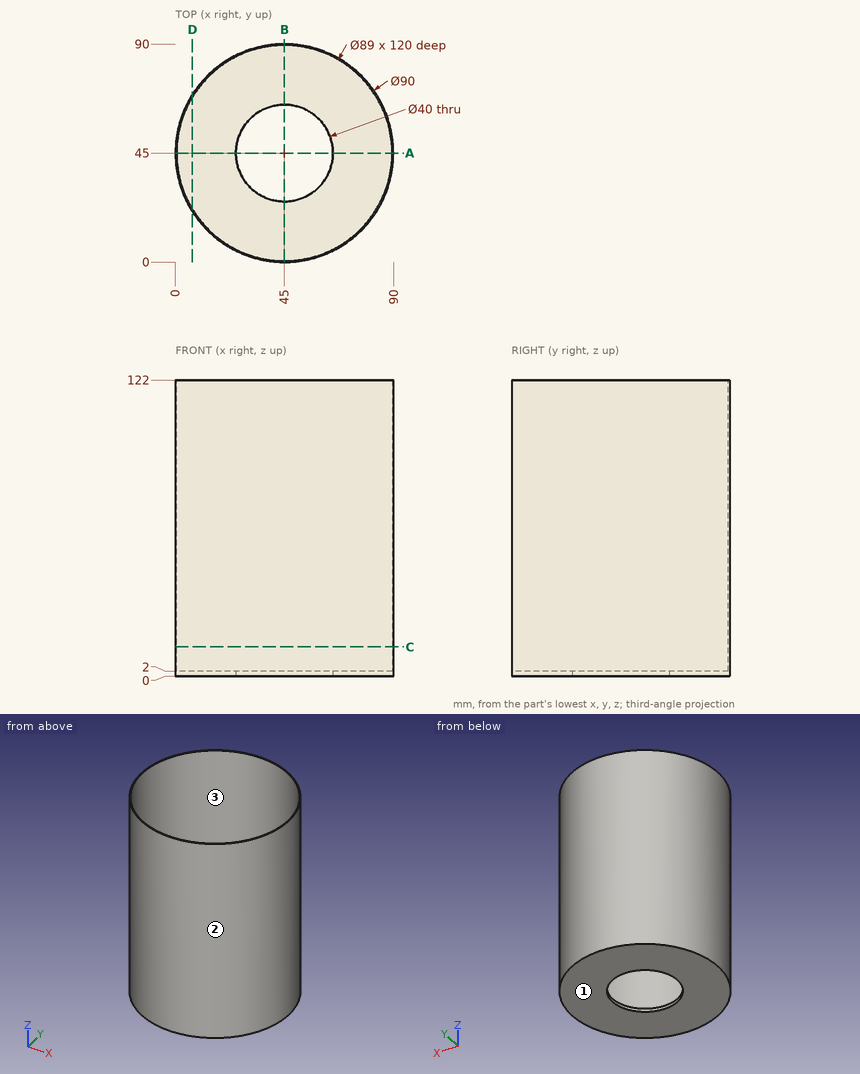
Print and shaded views of the part. All mm, measured from the part's lowest x, y and z. Round coordinates to 2 decimals unless told otherwise and drop trailing zeros. Write each loop counter-clockwise with the first axis right and the second up, starting at its lowest first coordinate (ties: lowest second). Pieces come first, ordered by that corner, then holes.
(1) Slice it at A-A, the plane y = 45. Write the cut outline in (x, z), and give its area (3 significant figures).
(2) Probe line 1 along Y through (x, z) = (45, 1); line 2 along Y through (x, z) = (71, 69); line 3 along X through (y, z) = (74, 75). List the from-to ranges inside material, lowest first.
(3) Slice it at D-D, the plane x = 7. Write the cut outline in (y, z), and give its area (3 significant figures).
(4) Slice it at C-C, the plane z = 12. Write the cut outline in (x, y), and give its area (3 significant figures).
(5) Drop flat-ended pins along their axis: P1, Ø12, axis at x = 26.5, y = 59.5, coming from the +Z side; P2, Ø1.5, axis at x = 65, z = 43.5, coming from the +Y side; P3, Ø10, axis at x = 59.5, z = 36.5, coming from the +Y side. Give the stop position or say it passes through.
(6) Mould opens along X. For the marked faces 1, 2 and 3 say: pulls with the +X half, pulls with the -X half, needs draft (parallel to the pull), parting line crosses it, or undercut.
From the geometry:
1. outline: (0, 0) - (25, 0) - (25, 2) - (0.5, 2) - (0.5, 122) - (0, 122) - close; (65, 0) - (90, 0) - (90, 122) - (89.5, 122) - (89.5, 2) - (65, 2) - close
1. area: 220 mm2
2. line 1: y = 0 to 25, 65 to 90
2. line 2: y = 8.27 to 8.89, 81.11 to 81.73
2. line 3: x = 10.59 to 11.25, 78.75 to 79.41
3. outline: (20.9, 0) - (69.1, 0) - (69.1, 122) - (68.16, 122) - (68.16, 2) - (21.84, 2) - (21.84, 122) - (20.9, 122) - close
3. area: 324 mm2
4. outline: circle Ø90 at (45, 45); hole circle Ø89 at (45, 45)
4. area: 141 mm2
5. P1: stops at z = 2
5. P2: stops at y = 85.67
5. P3: stops at y = 88.99
6. face 1: needs draft
6. face 2: parting line crosses it
6. face 3: undercut
